Part model, mm, in its own coordinate system. Give positions to 0.01 mm unless a question says otherwise; leave off trailing zeros. Order: outer loops, then holes, each group sorted by start corner. A loop starts at its lowest first (then second) coordinate and runs counter-clockwise, first axis right, second up. Notation, with made-up numbers: M 28.25,22.25 L 40.25,22.25 A20 ccw 40.25,30.25 Z; hole C 1.25,68.25 d8. An arc over 180 degrees is marked long. One line per question, with ' | ' between items.
```python
from build123d import *

# Parameters (mm, degrees)
SKETCH3_W           = 76.2
SKETCH3_H           = 9.525
BOSS_EXTRUDE1_DEPTH = 76.2
SKETCH4_R           = 3.5687
CUT_EXTRUDE2_DEPTH  = 86.725
CUT_EXTRUDE4_DEPTH  = 12.7
CUT_EXTRUDE6_DEPTH  = 12.7
CUT_EXTRUDE9_DEPTH  = 12.7
CUT_EXTRUDE10_DEPTH = 12.7


with BuildPart() as part:
    # Sketch3 → Boss-Extrude1 (new body)
    with BuildSketch(Plane.XY):
        Rectangle(SKETCH3_W, SKETCH3_H)
    extrude(amount=BOSS_EXTRUDE1_DEPTH)

    # Sketch4 → Cut-Extrude2 (cut, through all)
    with BuildSketch(Plane(origin=(0, 4.7625, 0), x_dir=(1, 0, 0), z_dir=(0, 1, 0))):
        with Locations(Location((0, -38.1, 0), (0, 0, 180))):
            Circle(SKETCH4_R)
    extrude(amount=-CUT_EXTRUDE2_DEPTH, mode=Mode.SUBTRACT)

    # Sketch5 → Cut-Extrude4 (cut)
    with BuildSketch(Plane(origin=(0, 4.7625, 0), x_dir=(1, 0, 0), z_dir=(0, 1, 0))):
        with BuildLine():
            Line((-38.1, -38.1), (-38.1, 0))
            Line((-38.1, 0), (0, 0))
            ThreePointArc((0, 0), (-26.940768363, -11.159231637), (-38.1, -38.1))
        make_face()
    extrude(amount=-CUT_EXTRUDE4_DEPTH, mode=Mode.SUBTRACT)

    # Sketch7 → Cut-Extrude6 (cut)
    with BuildSketch(Plane(origin=(0, 4.7625, 0), x_dir=(1, 0, 0), z_dir=(0, 1, 0))):
        with BuildLine():
            Line((0, 0), (38.1, 0))
            Line((38.1, 0), (38.1, -38.1))
            ThreePointArc((38.1, -38.1), (26.940768363, -11.159231637), (0, 0))
        make_face()
    extrude(amount=-CUT_EXTRUDE6_DEPTH, mode=Mode.SUBTRACT)

    # Sketch8 → Cut-Extrude9 (cut)
    with BuildSketch(Plane(origin=(0, 4.7625, 0), x_dir=(1, 0, 0), z_dir=(0, 1, 0))):
        with BuildLine():
            Line((38.1, -76.2), (38.1, -38.1))
            ThreePointArc((38.1, -38.1), (26.940768363, -65.040768363), (0, -76.2))
            Line((0, -76.2), (38.1, -76.2))
        make_face()
    extrude(amount=-CUT_EXTRUDE9_DEPTH, mode=Mode.SUBTRACT)

    # Sketch9 → Cut-Extrude10 (cut)
    with BuildSketch(Plane(origin=(0, 4.7625, 0), x_dir=(1, 0, 0), z_dir=(0, 1, 0))):
        with BuildLine():
            Line((0, -76.2), (-38.1, -76.2))
            Line((-38.1, -76.2), (-38.1, -38.1))
            ThreePointArc((-38.1, -38.1), (-26.940768363, -65.040768363), (0, -76.2))
        make_face()
    extrude(amount=-CUT_EXTRUDE10_DEPTH, mode=Mode.SUBTRACT)


solid = part.part
```
1. Slice it at C-C on z = 25.5. Give the cut face in (x, y), then the cut area to 3 significant figures.
Worked out:
outline: M -35.96,-4.76 L 35.96,-4.76 L 35.96,4.76 L -35.96,4.76 Z | area: 685 mm2
2. Slice it at B-B on x = -14. Give the cut face in (y, z), then the cut area to 3 significant figures.
Worked out:
outline: M -4.76,2.67 L 4.76,2.67 L 4.76,73.53 L -4.76,73.53 Z | area: 675 mm2
3. Probe L1, parallel to Z at x = 0, y = -1.25; L2, parallel to Z at x = 32, y = -2.25; L3, parallel to X at y = 3.5, z = 58.5. List the from-to ranges inside material, lowest first. Write a range as from..to.
Worked out:
L1: z = 0..34.53, 41.67..76.2 | L2: z = 17.42..58.78 | L3: x = -32.18..32.18
4. Mould opens along X. For faces 1 (the cylindrical face through (0.774, 0.067, 34.616)), 2 (the flat face through (-1, 4.762, 46)) say: released by +X, released by -X, zero draft, split by the parting line, or undercut.
Worked out:
face 1: undercut | face 2: zero draft
5. Drop flat-ended pins along their axis: pin 1 (4 mm diameter, centred on x = 30, y = -0.5, fed in from +Z); pin 2 (2 mm diameter, centred on x = 7, y = 2.5, fed in from +Z); pin 3 (4 mm diameter, centred on x = -5.5, y = -3, fed in from -Z); pin 4 (5.5 mm diameter, centred on x = 0, z = 38.1, fed in from -Y). Give the stop position or say it passes through.
Worked out:
pin 1: stops at z = 63.94 | pin 2: stops at z = 75.72 | pin 3: stops at z = 0.16 | pin 4: passes through
6. Slice it at A-A on y = 3.5. Give the cut face in (x, z).
Worked out:
outline: C 0,38.1 d76.2; hole C 0,38.1 d7.14
